Autodesk Inventor part; units mm, degrees
ref_plane "YZ Plane" through (0, 0, 0) normal (1, 0, 0) x (0, 1, 0)
ref_plane "XZ Plane" through (0, 0, 0) normal (0, 1, 0) x (-1, 0, 0)
ref_plane "XY Plane" through (0, 0, 0) normal (0, 0, 1) x (1, 0, 0)
sketch "Sketch1" plane through (0, 0, 0) normal (0, 0, 1) x (1, 0, 0)
  line L0 (-20.0958, 2.2922) -> (-2.5698, 2.2922)
  line L1 (-2.5698, 2.2922) -> (-2.5698, 6.2546)
  line L2 (-2.5698, 6.2546) -> (-7.3958, 6.2546)
  line L3 (-7.3958, 6.2546) -> (-7.3958, 4.6798)
  line L4 (-7.3958, 4.6798) -> (-20.0958, 4.6798)
  line L5 (-20.0958, 4.6798) -> (-20.0958, 2.2922)
  dimension "d0" = 12.7
  dimension "d1" = 2.3876
  dimension "d2" = 4.826
  dimension "d3" = 3.9624
revolve "Revolution1" add sketch "Sketch1" angle 360 about axis through (-20.0958, 2.2922, 0) along (1, 0, 0)
thread "Thread1"
sketch "Sketch2" plane through (-2.5698, 2.2922, 0) normal (1, 0, 0) x (0, 0, -1)
  circle A0 centre (0, 0) radius 3.9624
  line L0 (-1.3654, 1.8401) -> (0.9109, 2.1025)
  line L1 (0.9109, 2.1025) -> (2.2763, 0.2624)
  line L2 (2.2763, 0.2624) -> (1.3654, -1.8401)
  line L3 (1.3654, -1.8401) -> (-0.9109, -2.1025)
  line L4 (-0.9109, -2.1025) -> (-2.2763, -0.2624)
  line L5 (-2.2763, -0.2624) -> (-1.3654, 1.8401)
  dimension "d18" = 3.9688
extrude "Extrusion1" cut sketch "Sketch2" against normal blind 1.905 contours L0 L1 L2 L3 L4 L5
chamfer "Chamfer1" distance 0.254 angle 45 3 edges at (-2.5698, -1.6702, 0) (-7.3958, -1.6702, 0) (-20.0958, -0.0954, 0)
properties part number "HW-00070"
Verification items for the finished model (mm, model axes). A direction names the side the tool comes from. Give positions to 0.01 mm unless a question says otherwise; leave off trailing zeros. Order: outer loops, then holes, each group sorted by start corner. A loop starts at its lowest first (then second) coordinate and runs counter-clockwise, first axis right, second up. Notation, with made-up numbers: (-13.5, -19.5) -> (-3.5, -19.5) arc R18 cw to (-3.5, -10.5) -> close; hole circle Ø7 at (7.25, 48). An arc over 180 degrees is marked (long way). Use a Markdown table: item, result.
1) Depth check by flat-ended pin: pin 1 Ø1.5 at (x, y) = (-10, 2.5) entering from +Z; pin 2 Ø1 at (y, z) = (5.5, 1) entering from -X; pin 3 Ø3 at (x, z) = (-4.5, 3) entering from +Y. Enter the tip coordinate at first touch or a pass-through.
Results:
| item | result |
|---|---|
| pin 1 | z = 2.39 |
| pin 2 | x = -7.4 |
| pin 3 | y = 5.96 |
2) Section check B-B, the plane x = -14. Record the boundary of the cut face in (y, z), then the cut area to 3 significant figures.
Results:
| item | result |
|---|---|
| outline | circle Ø4.78 at (2.29, 0) |
| area | 17.9 mm² |
3) Mould release check, pull along Z, two halves, no side actions. Record for faces 1 (the flat face through (-3.509, 3.066, 1.827)), 2 (the flat face through (-7.396, 5, 0)), 3 (the cylindrical face through (-5.01, 1.78, -3.93)): pulls with the +Z half, pulls with the -Z half, needs draft (parallel to the pull), parting line crosses it, or undercut.
Results:
| item | result |
|---|---|
| face 1 | undercut |
| face 2 | needs draft |
| face 3 | parting line crosses it |
4) Material ranges on probe 1 along X at (y, z) = (3.5, 3.25); probe 2 along X at (y, z) = (0.5, 0); probe 3 along Y at (x, z) = (-6.25, 0.5), recorded low to high.
Results:
| item | result |
|---|---|
| probe 1 | -7.4 to -2.57 |
| probe 2 | -20.1 to -4.47 |
| probe 3 | -1.64 to 6.22 |
5) Section check A-A, the plane x = -6.75. Record the boundary of the cut face in (y, z).
Results:
| item | result |
|---|---|
| outline | circle Ø7.92 at (2.29, 0) |
6) Tool access check on faces 4 (the flat face through (-2.57, 4, -2)), 5 (the cylindrical face through (-13.71, 4.5, 0.91)), 6 (the flat face through (-3.509, 4.262, 0.243)). Record the directions out of +Z, -Z, +X, -X, +Y, -Y that give a thin tool (end or side, any length) a straight path to the whole face; none if there is none.
Results:
| item | result |
|---|---|
| face 4 | +Z, -Z, +X, +Y, -Y |
| face 5 | -X |
| face 6 | +X |
